Here's how the part is built. I have some questions about the finished solid (model axes, mm). A direction names the side the tool comes from. Give positions to 0.01 mm unless a question says otherwise; leave off trailing zeros. Write each loop counter-clockwise with the first axis right and the second up, starting at its lowest first coordinate (ties: lowest second). Pieces come first, ordered by that corner, then holes. Notation, with made-up numbers: (34.25, 87) - (72.25, 87) arc R6 ccw to (72.25, 92) - close; hole circle Ø11 at (36.25, 15.25). An arc over 180 degrees is marked (long way). Use a Markdown table: item, result.
```python
from build123d import *

# Parameters (mm, degrees)
SKETCH1_R           = 30
BOSS_EXTRUDE1_DEPTH = 220
SKETCH2_W           = 40
SKETCH2_H           = 60
CUT_EXTRUDE1_DEPTH  = 30
SKETCH3_R           = 2.5
CUT_EXTRUDE3_DEPTH  = 5
SKETCH4_W           = 5
SKETCH4_H           = 5
BOSS_EXTRUDE2_DEPTH = 31


with BuildPart() as part:
    # Sketch1 → Boss-Extrude1 (new body)
    with BuildSketch(Plane.XY):
        Circle(SKETCH1_R)
    extrude(amount=BOSS_EXTRUDE1_DEPTH)

    # Sketch2 → Cut-Extrude1 (cut)
    with BuildSketch(Plane.XY):
        Rectangle(SKETCH2_W, SKETCH2_H)
    extrude(amount=CUT_EXTRUDE1_DEPTH, mode=Mode.SUBTRACT)

    # Sketch3 → Cut-Extrude3 (cut)
    with BuildSketch(Plane.ZY.offset(-20)):
        with Locations((7.04424443, 0)):
            Circle(SKETCH3_R)
    cut_extrude3 = extrude(amount=-CUT_EXTRUDE3_DEPTH, mode=Mode.SUBTRACT)

    # Mirror1: Cut-Extrude3 across plane
    add(cut_extrude3.mirror(Plane.ZY), mode=Mode.SUBTRACT)

    # Sketch4 → Boss-Extrude2 (add)
    with BuildSketch(Plane(origin=(0, 0, 0), x_dir=(1, 0, 0), z_dir=(0, 1, 0))):
        with Locations((0, -217.5)):
            Rectangle(SKETCH4_W, SKETCH4_H)
    extrude(amount=BOSS_EXTRUDE2_DEPTH)


solid = part.part
```
Item 1: If we section it at C-C, the plane z = 42: Write out the boundary of the cut face in (x, y), plus the area to 3 significant figures.
Values:
| item | result |
|---|---|
| outline | circle Ø60 at (0, 0) |
| area | 2,830 mm2 |
Item 2: If we section it at D-D, the plane x = 11.5: Write out the boundary of the cut face in (y, z), plus the area to 3 significant figures.
Values:
| item | result |
|---|---|
| outline | (-27.71, 30) - (27.71, 30) - (27.71, 220) - (-27.71, 220) - close |
| area | 10,500 mm2 |
Item 3: I need wall thicknesses on line 1 along Z through (x, y) = (7, -10); line 2 along X through (y, z) = (4, 69.5); line 3 along Y through (x, z) = (-16.5, 73). Which ranges of each line are inside material? Lowest first, please. Write a range as [from, to].
Values:
| item | result |
|---|---|
| line 1 | z = [30, 220] |
| line 2 | x = [-29.73, 29.73] |
| line 3 | y = [-25.05, 25.05] |
Item 4: For faces 1 (the flat face through (0, 1, 220)), 2 (the cylindrical face through (22.46, 0.75, 9.43)), 3 (the flat face through (20, 0, 15)), which set-ups out of +Z, -Z, +X, -X, +Y, -Y let a thin tool reach every point of the face, with its end or its side?
Values:
| item | result |
|---|---|
| face 1 | +Z, +X, -X, +Y, -Y |
| face 2 | none |
| face 3 | -Z, +Y, -Y |
Item 5: Thinking about a two-plate mould opening in Z: for faces 4 (the flat face through (0, 31, 217)), 5 (the flat face through (0, 0, 30)), 6 (the cylindrical face through (-22.46, 0.75, 9.43)), which applies, +Z half, -Z half, draft (parallel to the pull), parting line (faces both ways), or undercut?
Values:
| item | result |
|---|---|
| face 4 | draft |
| face 5 | -Z half |
| face 6 | undercut |
Item 6: If we section it at A-A, the plane y = 0: Write out the boundary of the cut face in (x, z).
Values:
| item | result |
|---|---|
| outline | (-30, 0) - (-20, 0) - (-20, 4.54) - (-25, 4.54) - (-25, 9.54) - (-20, 9.54) - (-20, 30) - (20, 30) - (20, 9.54) - (25, 9.54) - (25, 4.54) - (20, 4.54) - (20, 0) - (30, 0) - (30, 220) - (-30, 220) - close |
Item 7: Will these pins go through, and if not, where does the flat tip stop? pin 1 Ø1.5 at (y, z) = (0.5, 6.5) entering from -X; pin 2 Ø2 at (x, z) = (-21, 151.5) entering from +Y; pin 3 Ø24 at (y, z) = (-2, 16) entering from +X; pin 4 Ø8 at (x, z) = (23, 136) entering from -Y.
Values:
| item | result |
|---|---|
| pin 1 | stops at x = -30 |
| pin 2 | stops at y = 22.36 |
| pin 3 | stops at x = 30 |
| pin 4 | stops at y = -23.22 |
Item 8: If we section it at B-B, the plane x = 0: Write out the boundary of the cut face in (y, z), plus the area to 3 significant figures.
Values:
| item | result |
|---|---|
| outline | (-30, 30) - (30, 30) - (30, 215) - (31, 215) - (31, 220) - (-30, 220) - close |
| area | 11,400 mm2 |
